from build123d import *

# Parameters (mm, degrees)
SKETCH1_W           = 58.8
SKETCH1_H           = 4
SKETCH1_W_2         = 4
SKETCH1_H_2         = 22
BOSS_EXTRUDE1_DEPTH = 11.5
CUT_EXTRUDE1_REACH  = 67.312
SKETCH2_R           = 1.65
SKETCH3_W           = 4
SKETCH3_H           = 26
BOSS_EXTRUDE2_DEPTH = 50
CUT_EXTRUDE2_REACH  = 80.607
SKETCH4_R           = 1.7
SKETCH4_W           = 20
SKETCH4_H           = 40.4
CHAMFER1_SIZE       = 10
FILLET1_R           = 2
FILLET2_R           = 2
FILLET3_R           = 2
FILLET4_R           = 2


with BuildPart() as part:
    # Sketch1 → Boss-Extrude1 (new body)
    with BuildSketch(Plane(origin=(0, 0, 0), x_dir=(1, 0, 0), z_dir=(0, 1, 0))):
        with Locations((29.4, -2)):
            Rectangle(SKETCH1_W, SKETCH1_H)
        with Locations((56.8, -15)):
            Rectangle(SKETCH1_W_2, SKETCH1_H_2)
    extrude(amount=BOSS_EXTRUDE1_DEPTH)

    # Sketch2 → Cut-Extrude1 (cut, up to next)
    with BuildSketch(Plane(origin=(0, 0, 0), x_dir=(-1, 0, 0), z_dir=(0, 0, -1)), mode=Mode.PRIVATE) as cut_extrude1_sk1:
        with Locations((-3.5, 5.75)):
            Circle(SKETCH2_R)
    cut_extrude1_tool1 = extrude(cut_extrude1_sk1.sketch, amount=-CUT_EXTRUDE1_REACH, mode=Mode.PRIVATE) & part.part
    # Sketch2 → Cut-Extrude1 (cut, up to next)
    with BuildSketch(Plane(origin=(0, 0, 0), x_dir=(-1, 0, 0), z_dir=(0, 0, -1)), mode=Mode.PRIVATE) as cut_extrude1_sk2:
        with Locations((-40.1, 5.75)):
            Circle(SKETCH2_R)
    cut_extrude1_tool2 = extrude(cut_extrude1_sk2.sketch, amount=-CUT_EXTRUDE1_REACH, mode=Mode.PRIVATE) & part.part
    add(cut_extrude1_tool1.solids().sort_by_distance((3.5, 5.75, 0))[0], mode=Mode.SUBTRACT)
    add(cut_extrude1_tool2.solids().sort_by_distance((40.1, 5.75, 0))[0], mode=Mode.SUBTRACT)

    # Sketch3 → Boss-Extrude2 (add)
    with BuildSketch(Plane.XZ):
        with Locations((56.8, 13)):
            Rectangle(SKETCH3_W, SKETCH3_H)
    extrude(amount=BOSS_EXTRUDE2_DEPTH)

    # Sketch4 → Cut-Extrude2 (cut, up to next)
    with BuildSketch(Plane.ZY.offset(-54.8), mode=Mode.PRIVATE) as cut_extrude2_sk1:
        with Locations((11, 5)):
            Circle(SKETCH4_R)
    cut_extrude2_tool1 = extrude(cut_extrude2_sk1.sketch, amount=-CUT_EXTRUDE2_REACH, mode=Mode.PRIVATE) & part.part
    # Sketch4 → Cut-Extrude2 (cut, up to next)
    with BuildSketch(Plane.ZY.offset(-54.8), mode=Mode.PRIVATE) as cut_extrude2_sk2:
        with Locations((21, 5)):
            Circle(SKETCH4_R)
    cut_extrude2_tool2 = extrude(cut_extrude2_sk2.sketch, amount=-CUT_EXTRUDE2_REACH, mode=Mode.PRIVATE) & part.part
    # Sketch4 → Cut-Extrude2 (cut, up to next)
    with BuildSketch(Plane.ZY.offset(-54.8), mode=Mode.PRIVATE) as cut_extrude2_sk3:
        with Locations((21, -45)):
            Circle(SKETCH4_R)
    cut_extrude2_tool3 = extrude(cut_extrude2_sk3.sketch, amount=-CUT_EXTRUDE2_REACH, mode=Mode.PRIVATE) & part.part
    # Sketch4 → Cut-Extrude2 (cut, up to next)
    with BuildSketch(Plane.ZY.offset(-54.8), mode=Mode.PRIVATE) as cut_extrude2_sk4:
        with Locations((11, -45)):
            Circle(SKETCH4_R)
    cut_extrude2_tool4 = extrude(cut_extrude2_sk4.sketch, amount=-CUT_EXTRUDE2_REACH, mode=Mode.PRIVATE) & part.part
    # Sketch4 → Cut-Extrude2 (cut, up to next)
    with BuildSketch(Plane.ZY.offset(-54.8), mode=Mode.PRIVATE) as cut_extrude2_sk5:
        with Locations((16, -20.2)):
            Rectangle(SKETCH4_W, SKETCH4_H)
    cut_extrude2_tool5 = extrude(cut_extrude2_sk5.sketch, amount=-CUT_EXTRUDE2_REACH, mode=Mode.PRIVATE) & part.part
    add(cut_extrude2_tool1.solids().sort_by_distance((54.8, 5, 11))[0], mode=Mode.SUBTRACT)
    add(cut_extrude2_tool2.solids().sort_by_distance((54.8, 5, 21))[0], mode=Mode.SUBTRACT)
    add(cut_extrude2_tool3.solids().sort_by_distance((54.8, -45, 21))[0], mode=Mode.SUBTRACT)
    add(cut_extrude2_tool4.solids().sort_by_distance((54.8, -45, 11))[0], mode=Mode.SUBTRACT)
    add(cut_extrude2_tool5.solids().sort_by_distance((54.8, -20.2, 16))[0], mode=Mode.SUBTRACT)

    # Chamfer1
    chamfer1_edges = [part.edges().sort_by_distance(p)[0] for p in [
        (54.8, 0, 2),
    ]]
    chamfer(chamfer1_edges, length=CHAMFER1_SIZE)

    # Fillet1
    fillet1_edges = [part.edges().sort_by_distance(p)[0] for p in [
        (54.8, 0.75, 4),
    ]]
    fillet(fillet1_edges, radius=FILLET1_R - 0.0001)  # a hair under: the kernel refuses the full size

    # Fillet2
    fillet2_edges = [part.edges().sort_by_distance(p)[0] for p in [
        (56.8, -50, 26),
        (56.8, -40.4, 26),
        (56.8, 0, 26),
        (56.8, 11.5, 26),
        (54.8, -10, 2.99995),
        (44.8, 0, 2),
        (0, 11.5, 2),
        (0, 0, 2),
    ]]
    fillet(fillet2_edges, radius=FILLET2_R)

    # Fillet3
    fillet3_edges = [part.edges().sort_by_distance(p)[0] for p in [
        (56.8, -40.4, 6),
        (56.8, 0, 6),
    ]]
    fillet(fillet3_edges, radius=FILLET3_R)

    # Fillet4
    fillet4_edges = [part.edges().sort_by_distance(p)[0] for p in [
        (56.8, -50, 0),
    ]]
    fillet(fillet4_edges, radius=FILLET4_R)


solid = part.part
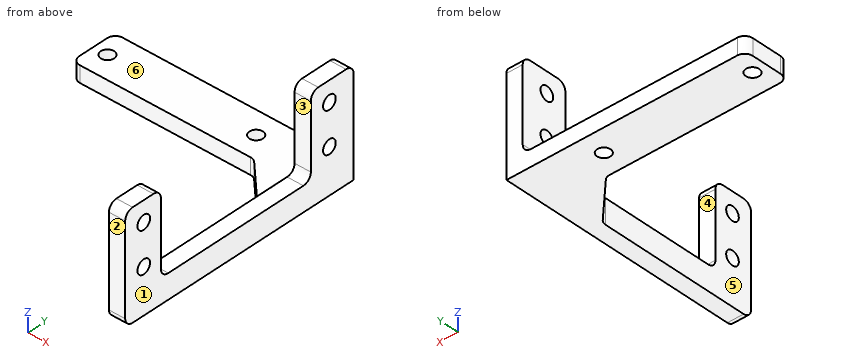
CAD build for the part. Positions are in the model's coordinates, mm. Face numbers are marked on the shaded views. A direction names the side the tool comes from. Coordinates: 2 decimals unless noted, no trailing zeros. Loops run counter-clockwise (first coordinate to the right, second up) from the corner with the lowest first, then second, coordinate; pieces in that order, holes last. Notation, with made-up numbers: (-23.5, 78) -> (27.5, 78) arc R12 ccw to (27.5, 84) -> close; hole circle Ø1 at (6, 34). An arc over 180 degrees is marked (long way). One line per item, written item: value.
1. Slice it at C-C on y = -45. Write the cut outline in (x, z).
Answers:
outline: (54.8, 0) -> (58.8, 0) -> (58.8, 9.3) -> (54.8, 9.3) -> close; (54.8, 12.7) -> (58.8, 12.7) -> (58.8, 19.3) -> (54.8, 19.3) -> close; (54.8, 22.7) -> (58.8, 22.7) -> (58.8, 26) -> (54.8, 26) -> close
2. Pull direction Y, two halves, no side cores. Call the marked faces 1, 2 and 3: pulls with the +Y half, pulls with the -Y half, needs draft (parallel to the pull), parting line crosses it, or undercut.
Answers:
face 1: needs draft
face 2: pulls with the -Y half
face 3: undercut
3. Slice it at B-B on z = 14.5. Write the cut outline in (x, y).
Answers:
outline: (54.8, -50) -> (58.8, -50) -> (58.8, -40.4) -> (54.8, -40.4) -> close; (54.8, 0) -> (58.8, 0) -> (58.8, 11.5) -> (54.8, 11.5) -> close
4. Flat gauge pins, fed straight in: P1, Ø5.5, axis at y = 5, z = 11, coming from the -X side; P2, Ø1.2, axis at x = 20, z = 1.5, coming from the -Y side; P3, Ø3, axis at x = 56, y = -24.5, coming from the +Z side. Where does each tip first touch, or does it go through?
Answers:
P1: stops at x = 54.8
P2: stops at y = 0
P3: stops at z = 6
5. Slice it at A-A on z = 11. Write the cut outline in (x, y).
Answers:
outline: (54.8, -50) -> (58.8, -50) -> (58.8, -46.7) -> (54.8, -46.7) -> close; (54.8, -43.3) -> (58.8, -43.3) -> (58.8, -40.4) -> (54.8, -40.4) -> close; (54.8, 0) -> (58.8, 0) -> (58.8, 3.3) -> (54.8, 3.3) -> close; (54.8, 6.7) -> (58.8, 6.7) -> (58.8, 11.5) -> (54.8, 11.5) -> close
6. Drill centre lines: line 1 (Y direction, x = 55.7, z = 11); line 2 (X direction, y = 4, z = 18.75); line 3 (Y direction, x = 6, z = 1.25). Where is each one in solid material? Low to high. Write a range as [from, to].
Answers:
line 1: y = [-50, -46.7], [-43.3, -40.4], [0, 3.3], [6.7, 11.5]
line 2: x = [54.8, 58.8]
line 3: y = [0, 11.5]
7. Which spindle directions (+Z, -Z, +X, -X, +Y, -Y) get a long thin tool onto all of the face, cutting with end or side? Do the marked faces 4, 5 and 6. Say none if no direction does.
Answers:
face 4: +Z, +X, -X
face 5: +Z, -X, -Y
face 6: +Z, -X, +Y, -Y
8. Slice it at D-D on x = 40.5. Write the cut outline in (y, z), and give its area (3 significant figures).
Answers:
outline: (0, 0) -> (4.15, 0) -> (4.15, 4) -> (0, 4) -> close; (7.35, 0) -> (11.5, 0) -> (11.5, 4) -> (7.35, 4) -> close
area: 33.2 mm^2
